```python
from build123d import *

# Parameters (mm, degrees)
SKETCH019_W     = 8.3
SKETCH019_H     = 3.35
PAD009_DEPTH    = 4.55
SKETCH020_W     = 0.6
SKETCH020_H     = 3.35
PAD010_DEPTH    = 0.6
SKETCH021_W     = 7.4
SKETCH021_H     = 2.45
POCKET005_DEPTH = 3.9
SKETCH022_W     = 6.9
SKETCH022_H     = 1.85
POCKET006_DEPTH = 0.45
SKETCH023_W     = 0.6
SKETCH023_H     = 0.6
PAD011_DEPTH    = 2.5
SKETCH024_W     = 0.6
SKETCH024_H     = 0.6
PAD012_DEPTH    = 3.75
SKETCH025_W     = 1.25
SKETCH025_H     = 2.95
POCKET007_DEPTH = 0.45


with BuildPart() as part:
    # Sketch019 → Pad009 (new body)
    with BuildSketch(Plane.XY):
        with Locations((4.15, 1.675)):
            Rectangle(SKETCH019_W, SKETCH019_H)
    extrude(amount=PAD009_DEPTH)

    # Sketch020 (on Face5 of Pad009) → Pad010 (join)
    with BuildSketch(Plane(origin=(0, 0, 0), x_dir=(1, 0, 0), z_dir=(0, 0, -1))):
        with Locations((0.3, -1.675)):
            Rectangle(SKETCH020_W, SKETCH020_H)
        with Locations((8, -1.675)):
            Rectangle(SKETCH020_W, SKETCH020_H)
    extrude(amount=PAD010_DEPTH)

    # Sketch021 (on Face7 of Pad010) → Pocket005 (cut)
    with BuildSketch(Plane.XY.offset(4.55)):
        with Locations((4.15, 1.675)):
            Rectangle(SKETCH021_W, SKETCH021_H)
    extrude(amount=-POCKET005_DEPTH, mode=Mode.SUBTRACT)

    # Sketch022 (on Face1 of Pocket005) → Pocket006 (cut)
    with BuildSketch(Plane.XZ):
        with Locations((4.15, 3.625)):
            Rectangle(SKETCH022_W, SKETCH022_H)
    extrude(amount=-POCKET006_DEPTH, mode=Mode.SUBTRACT)

    # Sketch023 (on Face3 of Pocket006) → Pad011 (join)
    with BuildSketch(Plane(origin=(0, 0, 0), x_dir=(1, 0, 0), z_dir=(0, 0, -1))):
        with Locations((1.76363, -2.15)):
            Rectangle(SKETCH023_W, SKETCH023_H)
        with Locations((3.01363, -2.15)):
            Rectangle(SKETCH023_W, SKETCH023_H)
        with Locations((4.26363, -2.15)):
            Rectangle(SKETCH023_W, SKETCH023_H)
        with Locations((5.51363, -2.15)):
            Rectangle(SKETCH023_W, SKETCH023_H)
        with Locations((6.76363, -2.15)):
            Rectangle(SKETCH023_W, SKETCH023_H)
    extrude(amount=PAD011_DEPTH)

    # Sketch024 (on Face3 of Pad011) → Pad012 (join)
    with BuildSketch(Plane(origin=(0, 0, 0), x_dir=(1, 0, 0), z_dir=(0, 0, -1))):
        with Locations((1.76363, -2.15)):
            Rectangle(SKETCH024_W, SKETCH024_H)
        with Locations((3.01363, -2.15)):
            Rectangle(SKETCH024_W, SKETCH024_H)
        with Locations((4.26363, -2.15)):
            Rectangle(SKETCH024_W, SKETCH024_H)
        with Locations((5.51363, -2.15)):
            Rectangle(SKETCH024_W, SKETCH024_H)
        with Locations((6.76363, -2.15)):
            Rectangle(SKETCH024_W, SKETCH024_H)
    extrude(amount=-PAD012_DEPTH)

    # Sketch025 (on Face14 of Pad012) → Pocket007 (cut)
    with BuildSketch(Plane(origin=(0, 3.35, 0), x_dir=(-1, 0, 0), z_dir=(0, 1, 0))):
        with Locations((-6.045, 1.475)):
            Rectangle(SKETCH025_W, SKETCH025_H)
        with Locations((-2.255, 1.475)):
            Rectangle(SKETCH025_W, SKETCH025_H)
    extrude(amount=-POCKET007_DEPTH, mode=Mode.SUBTRACT)


with BuildPart() as part_1:
    # Body002 placement: moved
    add(part.part.moved(Location((-3, -62, 126))))


solid = part_1.part
```
Can you work these out from the model? Positions are in its coordinate system, mm. A direction names the side the tool comes from. Round coordinates to 2 decimals unless told otherwise and drop trailing zeros. Loops run counter-clockwise (first coordinate to the right, second up) from the corner with the lowest first, then second, coordinate; pieces in that order, holes last.
Item 1: Please list where these lines run through material, in increasing order: L1, parallel to Y at x = -1.5, z = 127; L2, parallel to X at y = -60.9, z = 130; L3, parallel to Y at x = -2.5, z = 127.75.
Item 2: Suppose I cut it at D-D, the plane x = -1.75. Write out the boundary of the cut face in (y, z).
Item 3: Suppose I cut it at C-C, the plane y = -58.9. Write out the boundary of the cut face in (x, z), then the cut area to 3 significant figures.
Item 4: If we mould it in two halves opening along Y, with no side actions, what happens to faces 1 (the flat face through (-3, -60, 128)), 2 (the flat face through (1.1, -60.31, 126.65)), 3 (the flat face through (1, -62, 127))? For each: +Y half, -Y half, draft (parallel to the pull), parting line (faces both ways), or undercut.
Item 5: Suppose I cut it at A-A, the plane x = -0.5. Write out the boundary of the cut face in (y, z).
Item 6: Will these pins go through, and if not, where does the flat tip stop? pin 1 Ø0.7 at (x, y) = (4, -60) entering from +Z; pin 2 Ø1 at (x, y) = (-1.5, -61.5) entering from +Z; pin 3 Ø0.5 at (x, z) = (2.5, 125) entering from -Y.
Item 7: Which directions (+Z, -Z, +X, -X, +Y, -Y) give clear straight access to the entire face, cutting with the end or side of a thin tool? Please do faces 4 (the flat face through (5.3, -60, 128)), 5 (the flat face through (1, -59.1, 129)).
Item 8: Suppose I cut it at B-B, the plane z = 130.25. Write out the boundary of the cut face in (x, y).
Reported:
1. L1: y = -62 to -61.55, -60.15 to -59.55, -59.1 to -58.65
1. L2: x = -3 to -2.55, 4.85 to 5.3
1. L3: y = -62 to -61.55, -59.1 to -58.65
2. outline: (-62, 126) - (-58.65, 126) - (-58.65, 130.55) - (-59.1, 130.55) - (-59.1, 126.65) - (-61.55, 126.65) - (-61.55, 128.7) - (-62, 128.7) - close
3. outline: (-3, 125.4) - (-2.4, 125.4) - (-2.4, 126) - (-1.37, 126) - (-1.37, 128.95) - (-0.12, 128.95) - (-0.12, 126) - (2.42, 126) - (2.42, 128.95) - (3.67, 128.95) - (3.67, 126) - (4.7, 126) - (4.7, 125.4) - (5.3, 125.4) - (5.3, 130.55) - (-3, 130.55) - close
3. area: 31.1 mm2
4. face 1: draft
4. face 2: undercut
4. face 3: -Y half
5. outline: (-62, 126) - (-59.1, 126) - (-59.1, 126.65) - (-61.55, 126.65) - (-61.55, 128.7) - (-62, 128.7) - close; (-59.1, 128.95) - (-58.65, 128.95) - (-58.65, 130.55) - (-59.1, 130.55) - close
6. pin 1: stops at z = 129.75
6. pin 2: stops at z = 128.7
6. pin 3: stops at y = -60.15
7. face 4: +Z, -Z, +X, +Y, -Y
7. face 5: +Z
8. outline: (-3, -62) - (-2.3, -62) - (-2.3, -61.55) - (-2.55, -61.55) - (-2.55, -59.1) - (4.85, -59.1) - (4.85, -61.55) - (4.6, -61.55) - (4.6, -62) - (5.3, -62) - (5.3, -58.65) - (-3, -58.65) - close
